For this review, use the dimensioned drawing (mm, ordinates from the lowest corner) and the shaded views. A direction names the side the tool comes from. Give positions to 0.01 mm unless a question says otherwise; leave off trailing zeros. Order: outer loops, then holes, each group sorted by start corner. A loop starts at its lowest first (then second) coordinate and runs counter-clockwise, first axis right, second up. Notation, with made-up numbers: (-30.5, 24.5) - (19.5, 24.5) arc R14 cw to (19.5, 50.5) - close; hole circle Ø7 at (1, 32.25). An arc over 180 degrees is marked (long way). One line per item, written item: value.
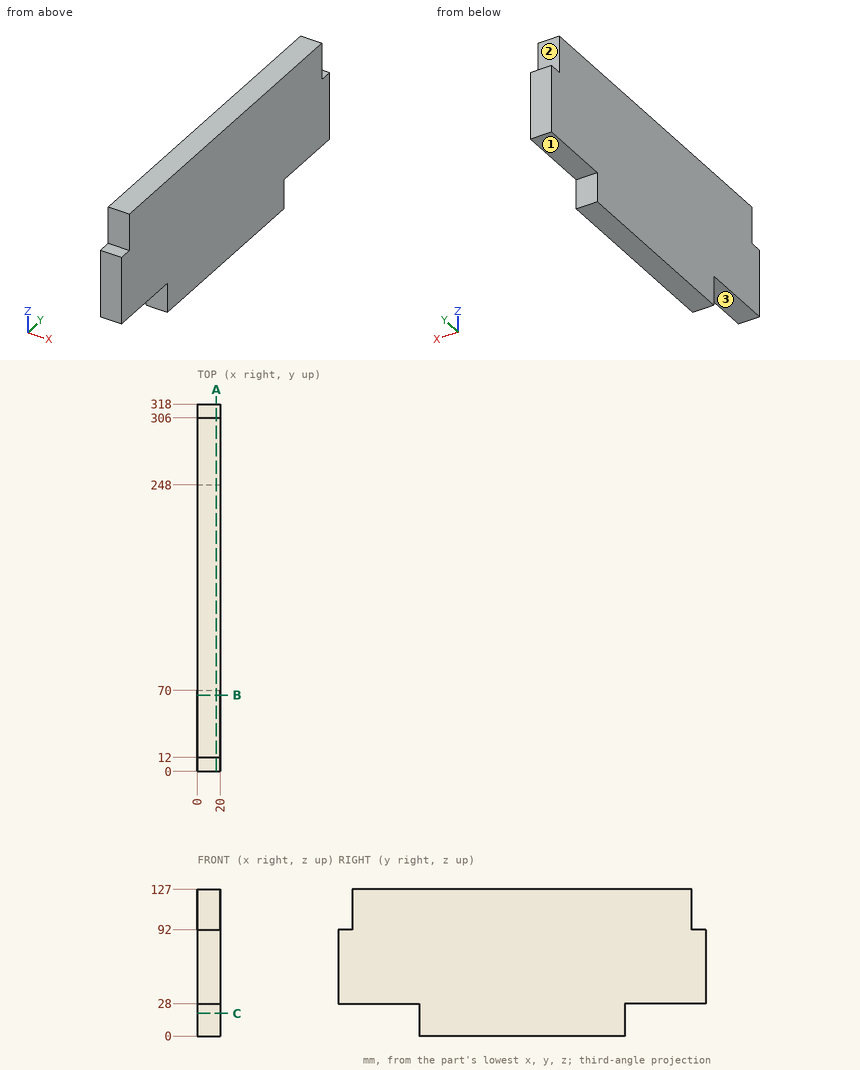
(1) Machinability: for the marked faces 1, 2 and 3, which of the approach directions +Z, -Z, +X, -X, +Y, -Y give a long, thin tool a straight path to every point of the face, cutting with its end or side? Answer none if there is none.
Answers below:
face 1: -Z, +X, -X, +Y
face 2: +Z, +X, -X, +Y
face 3: -Z, +X, -X, -Y
(2) Take a section at B-B (y = 66). Write out the cut boundary in (x, z), then the cut area to 3 significant figures.
Answers below:
outline: (0, 28) - (20, 28) - (20, 127) - (0, 127) - close
area: 1,980 mm^2
(3) For P1, Ø10, axis at x = 8.5, z = 112, coming from the -Y side; P2, Ø4, axis at x = 12.5, z = 109, coming from the +Y side; P3, Ø3.5, axis at x = 11.5, y = 314, coming from the +Z side, all flat-tipped, find the tip position at first contact; note any pin that passes through.
Answers below:
P1: stops at y = 12
P2: stops at y = 306
P3: stops at z = 92
(4) Take a section at C-C (z = 19.5). Write out the cut boundary in (x, y), then the cut area to 3 significant figures.
Answers below:
outline: (0, 70) - (20, 70) - (20, 248) - (0, 248) - close
area: 3,560 mm^2
(5) Wall thickness on line 1 (Y direction, x = 16.25, z = 105.5); line 2 (Z direction, x = 1, y = 31); line 3 (Y direction, x = 3.25, z = 9.5): over which ranges is each line inside the solid? List them lowest first. Write a range as from..to.
Answers below:
line 1: y = 12..306
line 2: z = 28..127
line 3: y = 70..248
(6) Take a section at A-A (x = 16.5). Write out the cut boundary in (y, z).
Answers below:
outline: (0, 28) - (70, 28) - (70, 0) - (248, 0) - (248, 28) - (318, 28) - (318, 92) - (306, 92) - (306, 127) - (12, 127) - (12, 92) - (0, 92) - close
